```python
from build123d import *

# Parameters (mm, degrees)
BOX_W           = 29
BOX_H           = 120
BOX_DEPTH       = 10
SKETCH_R        = 6
POCKET_DEPTH    = 10.001
SKETCH001_R     = 8
POCKET001_DEPTH = 5


with BuildPart() as part:
    # Box → Box (new body)
    with BuildSketch(Plane.XY):
        with Locations((14.5, 60)):
            Rectangle(BOX_W, BOX_H)
    extrude(amount=BOX_DEPTH)

    # Sketch → Pocket (cut, through all)
    with BuildSketch(Plane.XY.offset(10)):
        with Locations((12.5, 99.5)):
            Circle(SKETCH_R)
        with Locations((12.5, 20.5)):
            Circle(SKETCH_R)
    extrude(amount=-POCKET_DEPTH, mode=Mode.SUBTRACT)

    # Sketch001 → Pocket001 (cut)
    with BuildSketch(Plane.XY.offset(10)):
        with Locations((19.5, 60)):
            Circle(SKETCH001_R)
    extrude(amount=-POCKET001_DEPTH, mode=Mode.SUBTRACT)


solid = part.part
```
CAD build for the part. Positions are in the model's coordinates, mm. A direction names the side the tool comes from. Round coordinates to 2 decimals unless told otherwise and drop trailing zeros. Order: outer loops, then holes, each group sorted by start corner. A loop starts at its lowest first (then second) coordinate and runs counter-clockwise, first axis right, second up.
Item 1: Tool access for faces 1 (the face through (0, 59, 5)), 2 (the face through (19, 60, 5)): list every direction of +Z, -Z, +X, -X, +Y, -Y with a clear straight run to the whole face (end or side of a thin tool).
Item 2: Pin check, flat tip, straight feed: pin 1 (2 mm diameter, centred on x = 13, y = 16.5, fed in from -Z). Stop position of the tip, or through.
Item 3: Saw through at D-D on y = 60. Write the cut outline in (x, z), then the cut area to 3 significant figures.
Item 4: Saw through at A-A on y = 99.5. Write the cut outline in (x, z).
Item 5: Probe line 1 along Y through (x, z) = (12.75, 4); line 2 along Y through (x, z) = (19.5, 8.15); line 3 along Y through (x, z) = (11.25, 2). List the from-to ranges inside material, lowest first.
Item 6: Saw through at C-C on x = 10. Write the cut outline in (y, z), then the cut area to 3 significant figures.
Item 7: Saw through at B-B on z = 4. Write the cut outline in (x, y), then the cut area to 3 significant figures.
Item 8: Mould opens along X. For faces 3 (the face through (18.04, 18.2, 5.07)), 4 (the face through (29, 59, 5)), 5 (the face through (11, 61, 10)) say: pulls with the +X half, pulls with the -X half, needs draft (parallel to the pull), parting line crosses it, or undercut.
Reported:
1. face 1: +Z, -Z, -X, +Y, -Y
1. face 2: +Z
2. pin 1: passes through
3. outline: (0, 0) - (29, 0) - (29, 10) - (27.5, 10) - (27.5, 5) - (11.5, 5) - (11.5, 10) - (0, 10) - close
3. area: 210 mm2
4. outline: (0, 0) - (6.5, 0) - (6.5, 10) - (0, 10) - close; (18.5, 0) - (29, 0) - (29, 10) - (18.5, 10) - close
5. line 1: y = 0 to 14.51, 26.49 to 93.51, 105.49 to 120
5. line 2: y = 0 to 52, 68 to 120
5. line 3: y = 0 to 14.63, 26.37 to 93.63, 105.37 to 120
6. outline: (0, 0) - (15.05, 0) - (15.05, 10) - (0, 10) - close; (25.95, 0) - (94.05, 0) - (94.05, 10) - (25.95, 10) - close; (104.95, 0) - (120, 0) - (120, 10) - (104.95, 10) - close
6. area: 982 mm2
7. outline: (0, 0) - (29, 0) - (29, 120) - (0, 120) - close; hole circle Ø12 at (12.5, 20.5); hole circle Ø12 at (12.5, 99.5)
7. area: 3,250 mm2
8. face 3: undercut
8. face 4: pulls with the +X half
8. face 5: needs draft
